```python
from build123d import *

# Parameters (mm, degrees)
CHAMFER1_SIZE = 0.3


with BuildPart() as part:
    # Sketch1 → Revolve1 (revolve)
    with BuildSketch(Plane(origin=(0, 0, 0), x_dir=(0, 0, -1), z_dir=(1, 0, 0))):
        Polygon((4.75, 8.75), (-4.75, 8.75), (-4.75, 11), (-6.35, 11), (-6.35, 7.9875), (-1.55, 7.9875), (-1.55, 6.945), (1.55, 6.945), (1.55, 7.9875), (6.35, 7.9875), (6.35, 11), (4.75, 11), align=None)
    revolve(axis=Axis((0, 0, 0), (0, 0, -1)))

    # Chamfer1
    chamfer1_edges = [part.edges().sort_by_distance(p)[0] for p in [
        (0, -7.9875, 6.35),
        (0, -7.9875, -6.35),
    ]]
    chamfer(chamfer1_edges, length=CHAMFER1_SIZE)


solid = part.part
```
Source: CAD feature listing. Evaluate the final solid. Frame: model axes, mm. A direction names the side the tool comes from. Coordinates: 2 decimals unless noted, no trailing zeros. Loops run counter-clockwise (first coordinate to the right, second up) from the corner with the lowest first, then second, coordinate; pieces in that order, holes last. Notation, with made-up numbers: (59, 70.25) - (91, 70.25) arc R32 ccw to (91, 101.25) - close; hole circle Ø8 at (73.25, 17.5). An arc over 180 degrees is marked (long way). Answer as CSV lines item,"result".
1. Section D-D (x = 9.5). Return loops of the section in (y, z).
Established:
outline,"(-5.55, -6.35) - (5.55, -6.35) - (5.55, -4.75) - (-5.55, -4.75) - close; (-5.55, 4.75) - (5.55, 4.75) - (5.55, 6.35) - (-5.55, 6.35) - close"
2. Ray query, line 1 (Z direction, x = -1, y = 10); line 2 (X direction, y = 0, z = -4.35); line 3 (X direction, y = 0, z = -0.1) (3 decimals). Return the intervals inside material, ascending.
Established:
line 1,"z = -6.35 to -4.75, 4.75 to 6.35"
line 2,"x = -8.75 to -7.99, 7.99 to 8.75"
line 3,"x = -8.75 to -6.945, 6.945 to 8.75"
3. Contact query for flat-ended pins moving along their axis: pin 1 (4 mm diameter, centred on y = -5.5, z = -5, fed in from -X); pin 2 (1.5 mm diameter, centred on x = 0.5, z = 2.5, fed in from +Y); pin 3 (4 mm diameter, centred on y = -4.5, z = -3.5, fed in from +X); pin 4 (13 mm diameter, centred on x = 0, y = 0, fed in from -Z). Output: stop coordinate, or through.
Established:
pin 1,"stops at x = -10.43"
pin 2,"stops at y = 8.75"
pin 3,"stops at x = 10.6"
pin 4,"passes through"
4. Section C-C (z = -5.5). Return loops of the section in (x, y) (1 decimal).
Established:
outline,"circle Ø22 at (0, 0); hole circle Ø16 at (0, 0)"
5. Mould query, pull axis Z, two halves, no side actions, for faces 6 (the flat face through (7, -2, 1.55)), 7 (the cylindrical face through (-5.324, -6.944, 0.067)), 8 (the cylindrical face through (-6.78, -1.51, -0.02)), 9 (the flat face through (-9, 1, 4.75)). Classes: released by +Z, released by -Z, zero draft, split by the parting line, or undercut.
Established:
face 6,"released by +Z"
face 7,"undercut"
face 8,"zero draft"
face 9,"undercut"
6. Reachability of faces 1 (the flat face through (-9, -1, -4.75)), 2 (the cylindrical face through (-7.798, -1.732, 3.768)), 3 (the flat face through (7.4, -4.1, 6.35)), 4 (the cylindrical face through (-7.798, -1.732, -3.832)), 5 (the flat face through (7.4, 4.1, -6.35)) from +Z, -Z, +X, -X, +Y, -Y: full face, straight path, thin tool, end or side. Return the list, or none.
Established:
face 1,"none"
face 2,"+Z"
face 3,"+Z, +X, -X, +Y, -Y"
face 4,"-Z"
face 5,"-Z, +X, -X, +Y, -Y"
